Verification items for the finished model (mm, model axes). A direction names the side the tool comes from. Give positions to 0.01 mm unless a question says otherwise; leave off trailing zeros. Order: outer loops, then holes, each group sorted by start corner. A loop starts at its lowest first (then second) coordinate and runs counter-clockwise, first axis right, second up.
(1) Sectioned sample at D-D on x = -10. Record the cut outline in (y, z), plus the area to 3 significant figures.
(2) Sectioned sample at A-A on x = 10. Record the cut outline in (y, z).
(3) Gauge pin test, flat ends, axial feed: pin 1 (2 mm diameter, centred on x = 4, z = -6.5, fed in from +Y); pin 2 (5 mm diameter, centred on x = 0.5, y = 43, fed in from -Z). Record the tip position at first contact, or that the pin passes through.
(4) Sectioned sample at B-B on z = -3.75. Record the cut outline in (x, y), plus the area to 3 significant figures.
(5) Sectioned sample at C-C on z = 0. Record the cut outline in (x, y).
(6) Scan lines: L1, parallel to Y at x = 13, z = -7; L2, parallel to Y at x = -5, z = -9; L3, parallel to X at y = 39, z = 6.5. Record each from-to range of solid material in increasing order.
(7) Access from +Z, -Z, +X, -X, +Y, -Y to the whole of each face (thin tool, end or side, straight path). Record for faces 1 (the face through (12.49, 43.94, 0.55)), 2 (the face through (20, 20, 0)).
```python
from build123d import *

# Parameters (mm, degrees)
SKETCH_1_W      = 40
SKETCH_1_H      = 20
EXTRUDE_1_DEPTH = 40
SKETCH_2_R      = 2.55
EXTRUDE_2_DEPTH = 8
FILLET_1_R      = 2


with BuildPart() as part:
    # 草图1 → 凸台-拉伸1 (new body)
    with BuildSketch(Plane(origin=(0, 0, 0), x_dir=(1, 0, 0), z_dir=(0, 1, 0))):
        Rectangle(SKETCH_1_W, SKETCH_1_H)
    extrude(amount=EXTRUDE_1_DEPTH)

    # 草图2 → 凸台-拉伸2 (add)
    with BuildSketch(Plane(origin=(0, 40, 0), x_dir=(1, 0, 0), z_dir=(0, 1, 0))):
        with Locations(Location((10, 0, 0), (0, 0, 90))):
            Circle(SKETCH_2_R)
    extrude(amount=EXTRUDE_2_DEPTH)

    # 圆角1
    fillet_1_edges = [part.edges().sort_by_distance(p)[0] for p in [
        (-20, 40, 0),
        (0, 40, 10),
        (20, 40, 0),
        (0, 0, 10),
        (-20, 0, 0),
        (0, 0, -10),
        (20, 0, 0),
        (20, 20, 10),
        (-20, 20, 10),
        (-20, 20, -10),
        (20, 20, -10),
        (0, 40, -10),
    ]]
    fillet(fillet_1_edges, radius=FILLET_1_R)


solid = part.part
```
Ans:
1. outline: (0, -8) arc R2 ccw to (2, -10) - (38, -10) arc R2 ccw to (40, -8) - (40, 8) arc R2 ccw to (38, 10) - (2, 10) arc R2 ccw to (0, 8) - close
1. area: 797 mm2
2. outline: (0, -8) arc R2 ccw to (2, -10) - (38, -10) arc R2 ccw to (40, -8) - (40, -2.55) - (48, -2.55) - (48, 2.55) - (40, 2.55) - (40, 8) arc R2 ccw to (38, 10) - (2, 10) arc R2 ccw to (0, 8) - close
3. pin 1: stops at y = 40
3. pin 2: passes through
4. outline: (-20, 2) arc R2 ccw to (-18, 0) - (18, 0) arc R2 ccw to (20, 2) - (20, 38) arc R2 ccw to (18, 40) - (-18, 40) arc R2 ccw to (-20, 38) - close
4. area: 1,600 mm2
5. outline: (-20, 2) arc R2 ccw to (-18, 0) - (18, 0) arc R2 ccw to (20, 2) - (20, 38) arc R2 ccw to (18, 40) - (12.55, 40) - (12.55, 48) - (7.45, 48) - (7.45, 40) - (-18, 40) arc R2 ccw to (-20, 38) - close
6. L1: y = 0 to 40
6. L2: y = 0.27 to 39.73
6. L3: x = -19.73 to 19.73
7. face 1: +Y
7. face 2: +Z, -Z, +X, +Y, -Y
